from build123d import *
from build123d import SkipClean  # not in build123d's __all__

# Parameters (mm, degrees)
F0_R     = 68.5
F0_R_2   = 65.5
F1_DEPTH = 2
F2_DEPTH = 8.5
F3_SIZE  = 2
F5_DEPTH = 2
F6_DEPTH = 3
F7_DEPTH = 10
F8_DEPTH = 25
F9_R     = 2


# Not quite as in the source:
# - after a boolean that leaves OpenCascade's solid faulty, fix() repairs it


with BuildPart() as f1:
    # F0 (on Top) → F1 (new body)
    with BuildSketch(Plane.XY):
        Circle(F0_R)
        Circle(F0_R_2, mode=Mode.SUBTRACT)
        Circle(F0_R_2)
    extrude(amount=F1_DEPTH)

    # F0 (on Top) → F2 (join)
    with BuildSketch(Plane.XY):
        Circle(F0_R)
        Circle(F0_R_2, mode=Mode.SUBTRACT)
    extrude(amount=-F2_DEPTH)

    # F3
    f3_edges = [f1.edges().sort_by_distance(p)[0] for p in [
        (-68.5, 0, -8.5),
    ]]
    chamfer(f3_edges, length=F3_SIZE)

    # F4 (on Top) → F5 (join)
    with BuildSketch(Plane.XY):
        with BuildLine():
            Line((35, -74), (35, 49))
            ThreePointArc((35, 49), (31.7781745931, 56.7781745931), (24, 60))
            Line((24, 60), (-24, 60))
            ThreePointArc((-24, 60), (-31.7781745931, 56.7781745931), (-35, 49))
            Line((-35, 49), (-35, -74))
            ThreePointArc((-35, -74), (-31.7781745931, -81.7781745931), (-24, -85))
            Line((-24, -85), (24, -85))
            ThreePointArc((24, -85), (31.7781745931, -81.7781745931), (35, -74))
        make_face()
        with BuildLine():
            ThreePointArc((-32, 49), (-29.6568542495, 54.6568542495), (-24, 57))
            Line((-24, 57), (0, 57))
            Line((0, 57), (24, 57))
            ThreePointArc((24, 57), (29.6568542495, 54.6568542495), (32, 49))
            Line((32, 49), (32, -74))
            ThreePointArc((32, -74), (29.6568542495, -79.6568542495), (24, -82))
            Line((24, -82), (-24, -82))
            ThreePointArc((-24, -82), (-29.6568542495, -79.6568542495), (-32, -74))
            Line((-32, -74), (-32, 49))
        make_face(mode=Mode.SUBTRACT)
        with BuildLine():
            Line((0, 57), (-24, 57))
            ThreePointArc((-24, 57), (-29.6568542495, 54.6568542495), (-32, 49))
            Line((-32, 49), (-32, -74))
            ThreePointArc((-32, -74), (-29.6568542495, -79.6568542495), (-24, -82))
            Line((-24, -82), (24, -82))
            ThreePointArc((24, -82), (29.6568542495, -79.6568542495), (32, -74))
            Line((32, -74), (32, 49))
            ThreePointArc((32, 49), (29.6568542495, 54.6568542495), (24, 57))
            Line((24, 57), (0, 57))
        make_face()
    extrude(amount=-F5_DEPTH)

    # F4 (on Top) → F6 (cut)
    with BuildSketch(Plane.XY):
        with BuildLine():
            Line((0, 57), (-24, 57))
            ThreePointArc((-24, 57), (-29.6568542495, 54.6568542495), (-32, 49))
            Line((-32, 49), (-32, -74))
            ThreePointArc((-32, -74), (-29.6568542495, -79.6568542495), (-24, -82))
            Line((-24, -82), (24, -82))
            ThreePointArc((24, -82), (29.6568542495, -79.6568542495), (32, -74))
            Line((32, -74), (32, 49))
            ThreePointArc((32, 49), (29.6568542495, 54.6568542495), (24, 57))
            Line((24, 57), (0, 57))
        make_face()
    extrude(amount=F6_DEPTH, mode=Mode.SUBTRACT)

    # F4 (on Top) → F7 (join)
    with BuildSketch(Plane.XY):
        with BuildLine():
            Line((35, -74), (35, 49))
            ThreePointArc((35, 49), (31.7781745931, 56.7781745931), (24, 60))
            Line((24, 60), (-24, 60))
            ThreePointArc((-24, 60), (-31.7781745931, 56.7781745931), (-35, 49))
            Line((-35, 49), (-35, -74))
            ThreePointArc((-35, -74), (-31.7781745931, -81.7781745931), (-24, -85))
            Line((-24, -85), (24, -85))
            ThreePointArc((24, -85), (31.7781745931, -81.7781745931), (35, -74))
        make_face()
        with BuildLine():
            ThreePointArc((-32, 49), (-29.6568542495, 54.6568542495), (-24, 57))
            Line((-24, 57), (0, 57))
            Line((0, 57), (24, 57))
            ThreePointArc((24, 57), (29.6568542495, 54.6568542495), (32, 49))
            Line((32, 49), (32, -74))
            ThreePointArc((32, -74), (29.6568542495, -79.6568542495), (24, -82))
            Line((24, -82), (-24, -82))
            ThreePointArc((-24, -82), (-29.6568542495, -79.6568542495), (-32, -74))
            Line((-32, -74), (-32, 49))
        make_face(mode=Mode.SUBTRACT)
    with SkipClean():  # cleaning this boolean's faces spoils the solid; the shape is the same uncleaned
        extrude(amount=F7_DEPTH)

    # F0 (on Top) → F8 (cut)
    with BuildSketch(Plane.XY):
        Circle(F0_R_2)
    extrude(amount=-F8_DEPTH, mode=Mode.SUBTRACT)

    add(f1.part.fix(), mode=Mode.REPLACE)

    # F9
    f9_edges = [f1.edges().sort_by_distance(p)[0] for p in [
        (-33.872924, 59.538853, 2),
    ]]
    fillet(f9_edges, radius=F9_R)


solid = f1.part
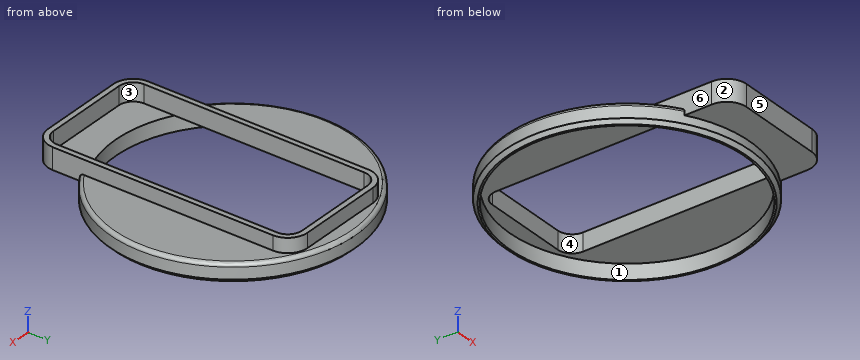
Design review of the part built by this model. Coordinates are the model's own, in mm. Face numbers are marked on the shaded views. A direction names the side the tool comes from. Give positions to 0.01 mm unless a question says otherwise; leave off trailing zeros. Loops run counter-clockwise (first coordinate to the right, second up) from the corner with the lowest first, then second, coordinate; pieces in that order, holes last. Notation, with made-up numbers: M -28,42 L 9,42 A13 ccw 9,49 Z; hole C -32.5,-36.75 d3. An arc over 180 degrees is marked long. Write item = value, one per line.
Q1. Draft analysis for pull direction Y (two halves, no side actions). For the marked faces 4, 5 and 6, state which applies: +Y half, -Y half, draft (parallel to the pull), parting line (faces both ways), or undercut.
Output values:
face_4 = undercut
face_5 = -Y half
face_6 = draft
Q2. We need section B-B (x = 0). Give the boundary of the cut face in (y, z), plus the area to 3 significant figures.
Output values:
outline = M -85,-2 L -68.5,-2 L -68.5,-6.5 L -66.5,-8.5 L -65.5,-8.5 L -65.5,0 L -82,0 L -82,10 L -85,10 Z; M 57,0 L 65.5,0 L 65.5,-8.5 L 66.5,-8.5 L 68.5,-6.5 L 68.5,0 A2 ccw 66.5,2 L 60,2 L 60,10 L 57,10 Z
area = 156 mm^2
Q3. We need section D-D (z = -3.75). Give the boundary of the cut face in (x, y).
Output values:
outline = C 0,0 d137; hole C 0,0 d131
Q4. Insertion check: pin 1 (6 mm diameter, centred on y = -23, z = 4.5, fed in from -X); pin 2 (1 mm diameter, centred on x = 47, z = -3, fed in from -Y); pin 3 (5 mm diameter, centred on y = -42, z = -6.5, fed in from +X). Each pin has a flat end and moves straight along its axis. Give the tip position at first contact, or say it passes through.
Output values:
pin_1 = -63.95
pin_2 = -50.3
pin_3 = 55.96
Q5. To check wall thickness, follow line 1 (X direction, y = -1, z = 3); line 2 (X direction, y = 0, z = -2.5). State the ranges of each line that lie inside material, in increasing order. Write a range as [from, to].
Output values:
line_1 = [-35, -32], [32, 35]
line_2 = [-68.5, -65.5], [65.5, 68.5]
Q6. We need section A-A (z = 5.25). Give the boundary of the cut face in (x, y), plus the area to 3 significant figures.
Output values:
outline = M -35,-74 A11 ccw -24,-85 L 24,-85 A11 ccw 35,-74 L 35,49 A11 ccw 24,60 L -24,60 A11 ccw -35,49 Z; hole M -32,-74 A8 ccw -24,-82 L 24,-82 A8 ccw 32,-74 L 32,49 A8 ccw 24,57 L -24,57 A8 ccw -32,49 Z
area = 1,210 mm^2
Q7. For the marked faces 1, 2 and 3, list the 3-axis set-ups (+Z, -Z, +X, -X, +Y, -Y) from which the entire face can be reached by the end or side of a thin tool; tool diameter is ignored.
Output values:
face_1 = -Z
face_2 = +Z, -Z, -X, -Y
face_3 = +Z
Q8. We need section C-C (y = 0). Give the boundary of the cut face in (x, z), plus the area to 3 significant figures.
Output values:
outline = M -68.5,-6.5 L -66.5,-8.5 L -65.5,-8.5 L -65.5,0 L -32,0 L -32,10 L -35,10 L -35,2 L -66.5,2 A2 ccw -68.5,0 Z; M 32,0 L 65.5,0 L 65.5,-8.5 L 66.5,-8.5 L 68.5,-6.5 L 68.5,0 A2 ccw 66.5,2 L 35,2 L 35,10 L 32,10 Z
area = 239 mm^2
